```python
from build123d import *

# Parameters (mm, degrees)
F2_R     = 1.85
F3_DEPTH = 11.251
F4_R     = 2.25
F4_R_2   = 11.25
F4_R_3   = 10.75
F5_DEPTH = 2


with BuildPart() as f1:
    # F0 (on Right) → F1 (revolve)
    with BuildSketch(Plane.YZ):
        Polygon((11.5, 11.25), (0, 11.25), (0, 10.75), (7, 10.75), (7, 10), (10.5, 10), (10.5, 1.9), (11.5, 1.9), (11.5, 4), (19.5, 4), (19.5, 4.7), (11.5, 4.7), align=None)
    revolve(axis=Axis((0, 13.454885, 0), (0, 1, 0)))

    # F2 (on Top) → F3 (cut, through all)
    with BuildSketch(Plane.XY):
        with Locations((0, 2.5)):
            Circle(F2_R)
    extrude(amount=-F3_DEPTH, mode=Mode.SUBTRACT)

    # F4 (on face) → F5 (join)
    with BuildSketch(Plane(origin=(0, 11.5, 0), x_dir=(-1, 0, 0), z_dir=(0, 1, 0))):
        with BuildLine():
            Line((17.320508, -5), (4.330127, 17.5))
            ThreePointArc((4.330127, 17.5), (0, 20), (-4.330127, 17.5))
            Line((-4.330127, 17.5), (-17.320508, -5))
            ThreePointArc((-17.320508, -5), (-17.320508, -10), (-12.990381, -12.5))
            Line((-12.990381, -12.5), (12.990381, -12.5))
            ThreePointArc((12.990381, -12.5), (17.320508, -10), (17.320508, -5))
        make_face()
        with Locations((-12.990381, -7.5)):
            Circle(F4_R, mode=Mode.SUBTRACT)
        Circle(F4_R_2, mode=Mode.SUBTRACT)
        with Locations((12.990381, -7.5)):
            Circle(F4_R, mode=Mode.SUBTRACT)
        with Locations((0, 15)):
            Circle(F4_R, mode=Mode.SUBTRACT)
        Circle(F4_R_2)
        Circle(F4_R_3, mode=Mode.SUBTRACT)
    extrude(amount=-F5_DEPTH)


solid = f1.part
```
Input: part model. Units: mm. Frame: model coordinates. A direction names the side the tool comes from. Coordinates: 2 decimals unless noted, no trailing zeros. Loops run counter-clockwise (first coordinate to the right, second up) from the corner with the lowest first, then second, coordinate; pieces in that order, holes last.
Q1. Set-up query: faces 1 (the cylindrical face through (-17.283, 10.514, -10.063)), 2 (the cylindrical face through (-9.76, 8.77, -2.17)), 3 (the cylindrical face through (-4.59, 15.44, -1.02)). Return all of +Z, -Z, +X, -X, +Y, -Y with unobstructed straight access to the full face (end or side cutting, diameter ignored); none if empty.
Results are:
face 1: -X, +Y, -Y
face 2: -Y
face 3: +Y
Q2. Section B-B, the plane z = -0.5. Return the cut outline in (x, y), and give its area (3 significant figures).
Results are:
outline: (-14.72, 9.5) - (-11.24, 9.5) - (-11.24, 0) - (-10.74, 0) - (-10.74, 7) - (-9.99, 7) - (-9.99, 10.5) - (-1.83, 10.5) - (-1.83, 11.5) - (-3.97, 11.5) - (-3.97, 19.5) - (-4.67, 19.5) - (-4.67, 11.5) - (-14.72, 11.5) - close; (1.83, 10.5) - (9.99, 10.5) - (9.99, 7) - (10.74, 7) - (10.74, 0) - (11.24, 0) - (11.24, 9.5) - (14.72, 9.5) - (14.72, 11.5) - (4.67, 11.5) - (4.67, 19.5) - (3.97, 19.5) - (3.97, 11.5) - (1.83, 11.5) - close
area: 59.8 mm2
Q3. Mould query, pull axis Y, two halves, no side actions, for faces 4 (the cylindrical face through (-1.468, 1.374, -10.914)), 5 (the flat face through (4, 19.5, -2)), 6 (the flat face through (-10.92, 10.51, 6.09)). Classes: +Y half, -Y half, draft (parallel to the pull), parting line (faces both ways), or undercut.
Results are:
face 4: undercut
face 5: +Y half
face 6: draft
Q4. Section C-C, the plane y = 13.75. Return the cut outline in (x, z), and give its area (3 significant figures).
Results are:
outline: circle Ø9.4 at (0, 0); hole circle Ø8 at (0, 0)
area: 19.1 mm2
Q5. Section D-D, the plane x = 0. Give the number of separate pieces and of enclosed holes in the cut face, and give its area (3 significant figures).
Results are:
separate pieces: 4
enclosed holes: 0
area: 54.8 mm2
Q6. Line query: line 1 along X through (y, z) = (6, 0.5); line 2 along X through (y, z) = (17.5, 0); line 3 along Y through (x, z) = (-4, -6.5). Output: solid intervals per line, ascending.
Results are:
line 1: x = -11.24 to -10.74, 10.74 to 11.24
line 2: x = -4.7 to -4, 4 to 4.7
line 3: y = 10.5 to 11.5
Q7. Section A-A, the plane z = -7.5. Return the cut outline in (x, y), and give its area (3 significant figures).
Results are:
outline: (-17.99, 9.5) - (-15.24, 9.5) - (-15.24, 11.5) - (-17.99, 11.5) - close; (-10.74, 9.5) - (-8.39, 9.5) - (-8.39, 0) - (-7.7, 0) - (-7.7, 7) - (-6.61, 7) - (-6.61, 10.5) - (6.61, 10.5) - (6.61, 7) - (7.7, 7) - (7.7, 0) - (8.39, 0) - (8.39, 9.5) - (10.74, 9.5) - (10.74, 11.5) - (-10.74, 11.5) - close; (15.24, 9.5) - (17.99, 9.5) - (17.99, 11.5) - (15.24, 11.5) - close
area: 59.2 mm2
Q8. Contact query for flat-ended pins moving along their axis: pin 1 (5 mm diameter, centred on x = 0, y = 2.5, fed in from +Z); pin 2 (5 mm diameter, centred on x = 0, z = 15, fed in from -Y); pin 3 (11 mm diameter, centred on x = -2.5, z = 1.5, fed in from -Y). Output: stop coordinate, or through.
Results are:
pin 1: stops at z = 11.25
pin 2: stops at y = 9.5
pin 3: stops at y = 10.5
